Source: CAD feature listing. Evaluate the final solid. Frame: model axes, mm. A direction names the side the tool comes from. Round coordinates to 2 decimals unless told otherwise and drop trailing zeros. Loops run counter-clockwise (first coordinate to the right, second up) from the corner with the lowest first, then second, coordinate; pieces in that order, holes last. Notation, with made-up numbers: (-21, 42.5) - (-1, 42.5) arc R13 ccw to (-1, 48.5) - close; hole circle Ø3 at (-25.75, -17.75). An arc over 180 degrees is marked (long way). One line per question, with ' | ' between items.
from build123d import *

# Parameters (mm, degrees)
SKETCH1_R           = 66
SKETCH1_R_2         = 54
BOSS_EXTRUDE1_DEPTH = 30
SKETCH2_R           = 1.45
CUT_EXTRUDE1_DEPTH  = 5
BOSS_EXTRUDE2_START = 3
SKETCH3_R           = 66
BOSS_EXTRUDE2_DEPTH = 3
SKETCH4_R           = 11
SKETCH4_R_2         = 2.45
CUT_EXTRUDE2_DEPTH  = 99.04080783


with BuildPart() as part:
    # Sketch1 → Boss-Extrude1 (new body)
    with BuildSketch(Plane(origin=(0, 0, 0), x_dir=(1, 0, 0), z_dir=(0, 1, 0))):
        with Locations(Location((0, 0, 0), (0, 0, 270))):
            Circle(SKETCH1_R)
        with Locations(Location((0, 0, 0), (0, 0, 270))):
            Circle(SKETCH1_R_2, mode=Mode.SUBTRACT)
    extrude(amount=BOSS_EXTRUDE1_DEPTH)

    # Sketch2 → Cut-Extrude1 (cut)
    with BuildSketch(Plane(origin=(0, 30, 0), x_dir=(1, 0, 0), z_dir=(0, 1, 0))):
        with Locations(Location((0, 60, 0), (0, 0, 270))):
            Circle(SKETCH2_R)
        with Locations(Location((11.705419321, 58.847116824, 0), (0, 0, 270))):
            Circle(SKETCH2_R)
        with Locations(Location((22.961005942, 55.432771951, 0), (0, 0, 270))):
            Circle(SKETCH2_R)
        with Locations(Location((33.334213981, 49.888176738, 0), (0, 0, 270))):
            Circle(SKETCH2_R)
        with Locations(Location((42.426406871, 42.426406871, 0), (0, 0, 270))):
            Circle(SKETCH2_R)
        with Locations(Location((49.888176738, 33.334213981, 0), (0, 0, 270))):
            Circle(SKETCH2_R)
        with Locations(Location((55.432771951, 22.961005942, 0), (0, 0, 270))):
            Circle(SKETCH2_R)
        with Locations(Location((58.847116824, 11.705419321, 0), (0, 0, 270))):
            Circle(SKETCH2_R)
        with Locations(Location((60, 0, 0), (0, 0, 270))):
            Circle(SKETCH2_R)
        with Locations(Location((58.847116824, -11.705419321, 0), (0, 0, 270))):
            Circle(SKETCH2_R)
        with Locations(Location((55.432771951, -22.961005942, 0), (0, 0, 270))):
            Circle(SKETCH2_R)
        with Locations(Location((49.888176738, -33.334213981, 0), (0, 0, 270))):
            Circle(SKETCH2_R)
        with Locations(Location((42.426406871, -42.426406871, 0), (0, 0, 270))):
            Circle(SKETCH2_R)
        with Locations(Location((33.334213981, -49.888176738, 0), (0, 0, 270))):
            Circle(SKETCH2_R)
        with Locations(Location((22.961005942, -55.432771951, 0), (0, 0, 270))):
            Circle(SKETCH2_R)
        with Locations(Location((11.705419321, -58.847116824, 0), (0, 0, 270))):
            Circle(SKETCH2_R)
        with Locations(Location((0, -60, 0), (0, 0, 270))):
            Circle(SKETCH2_R)
        with Locations(Location((-11.705419321, -58.847116824, 0), (0, 0, 270))):
            Circle(SKETCH2_R)
        with Locations(Location((-22.961005942, -55.432771951, 0), (0, 0, 270))):
            Circle(SKETCH2_R)
        with Locations(Location((-33.334213981, -49.888176738, 0), (0, 0, 270))):
            Circle(SKETCH2_R)
        with Locations(Location((-42.426406871, -42.426406871, 0), (0, 0, 270))):
            Circle(SKETCH2_R)
        with Locations(Location((-49.888176738, -33.334213981, 0), (0, 0, 270))):
            Circle(SKETCH2_R)
        with Locations(Location((-55.432771951, -22.961005942, 0), (0, 0, 270))):
            Circle(SKETCH2_R)
        with Locations(Location((-58.847116824, -11.705419321, 0), (0, 0, 270))):
            Circle(SKETCH2_R)
        with Locations(Location((-60, 0, 0), (0, 0, 270))):
            Circle(SKETCH2_R)
        with Locations(Location((-58.847116824, 11.705419321, 0), (0, 0, 270))):
            Circle(SKETCH2_R)
        with Locations(Location((-55.432771951, 22.961005942, 0), (0, 0, 270))):
            Circle(SKETCH2_R)
        with Locations(Location((-49.888176738, 33.334213981, 0), (0, 0, 270))):
            Circle(SKETCH2_R)
        with Locations(Location((-42.426406871, 42.426406871, 0), (0, 0, 270))):
            Circle(SKETCH2_R)
        with Locations(Location((-33.334213981, 49.888176738, 0), (0, 0, 270))):
            Circle(SKETCH2_R)
        with Locations(Location((-22.961005942, 55.432771951, 0), (0, 0, 270))):
            Circle(SKETCH2_R)
        with Locations(Location((-11.705419321, 58.847116824, 0), (0, 0, 270))):
            Circle(SKETCH2_R)
    extrude(amount=-CUT_EXTRUDE1_DEPTH, mode=Mode.SUBTRACT)

    # Sketch3 → Boss-Extrude2 (add)
    with BuildSketch(Plane.XZ.offset(BOSS_EXTRUDE2_START)):
        with Locations(Location((0, 0, 0), (0, 0, 270))):
            Circle(SKETCH3_R)
    extrude(amount=-BOSS_EXTRUDE2_DEPTH)

    # Sketch4 → Cut-Extrude2 (cut, through all)
    with BuildSketch(Plane(origin=(0, 0, 0), x_dir=(1, 0, 0), z_dir=(0, 1, 0))):
        with Locations(Location((0, 0, 0), (0, 0, 270))):
            Circle(SKETCH4_R)
        with Locations(Location((0, 17.45, 0), (0, 0, 270))):
            Circle(SKETCH4_R_2)
        with Locations(Location((-15.112143296, -8.725, 0), (0, 0, 270))):
            Circle(SKETCH4_R_2)
        with Locations(Location((15.112143296, -8.725, 0), (0, 0, 270))):
            Circle(SKETCH4_R_2)
    extrude(amount=-CUT_EXTRUDE2_DEPTH, mode=Mode.SUBTRACT)


solid = part.part
1. Contact query for flat-ended pins moving along their axis: P1, Ø1.4, axis at x = -22.5, z = -55, coming from the +Y side; P2, Ø2, axis at y = 1, z = -0.5, coming from the +X side; P3, Ø3, axis at x = 44.5, z = 3.5, coming from the +Y side; P4, Ø2.5, axis at x = -60, z = 0.5, coming from the +Y side. Output: stop coordinate, or through.
Worked out:
P1: stops at y = 25 | P2: stops at x = 66 | P3: stops at y = 0 | P4: stops at y = 30
2. Section query B-B, the plane z = 8. Return loops of the section in (x, y), plus the area to 3 significant figures.
Worked out:
outline: (-65.51, -3) - (-17.45, -3) - (-17.45, 0) - (-53.4, 0) - (-53.4, 30) - (-65.51, 30) - close; (-12.77, -3) - (-7.55, -3) - (-7.55, 0) - (-12.77, 0) - close; (7.55, -3) - (12.77, -3) - (12.77, 0) - (7.55, 0) - close; (17.45, -3) - (65.51, -3) - (65.51, 30) - (53.4, 30) - (53.4, 0) - (17.45, 0) - close | area: 1,050 mm2
3. Access query for faces 1 (the cylindrical face through (0.108, -1.479, -19.898)), 2 (the flat face through (-33, 25, -50)). Directions: +Z, -Z, +X, -X, +Y, -Y. A direction counts if a zero-diameter tool reaches every point of the face in a straight line with its end or side. Return the directions, or none.
Worked out:
face 1: +Y, -Y | face 2: +Y
4. Section query D-D, the plane z = -17.45. Return loops of the section in (x, y).
Worked out:
outline: (-63.65, -3) - (-2.45, -3) - (-2.45, 0) - (-51.1, 0) - (-51.1, 30) - (-63.65, 30) - close; (2.45, -3) - (63.65, -3) - (63.65, 30) - (51.1, 30) - (51.1, 0) - (2.45, 0) - close
5. Section query A-A, the plane x = 6. Return loops of the section in (y, z), plus the area to 3 significant figures.
Worked out:
outline: (-3, -65.73) - (30, -65.73) - (30, -53.67) - (0, -53.67) - (0, -9.22) - (-3, -9.22) - close; (-3, 9.22) - (0, 9.22) - (0, 53.67) - (30, 53.67) - (30, 65.73) - (-3, 65.73) - close | area: 1,060 mm2
6. Section query C-C, the plane y = 20. Return loops of the section in (x, z).
Worked out:
outline: circle Ø132 at (0, 0); hole circle Ø108 at (0, 0)
7. Mould query, pull axis X, two halves, no side actions, for faces 3 (the flat face through (54, 30, -5)), 4 (the cylindrical face through (56.87, 27.54, -23.15)). Classes: released by +X, released by -X, zero draft, split by the parting line, or undercut.
Worked out:
face 3: zero draft | face 4: undercut
8. Material intervals for probe 1 along X at (y, z) = (28.5, 41.5); probe 2 along Y at (x, z) = (-33.5, -16); probe 3 along X at (y, z) = (27, 22), sorted ascending.
Worked out:
probe 1: x = -51.32 to -43.54, -41.31 to -34.55, 34.55 to 41.31, 43.54 to 51.32 | probe 2: y = -3 to 0 | probe 3: x = -62.23 to -56.52, -54.35 to -49.32, 49.32 to 54.35, 56.52 to 62.23
